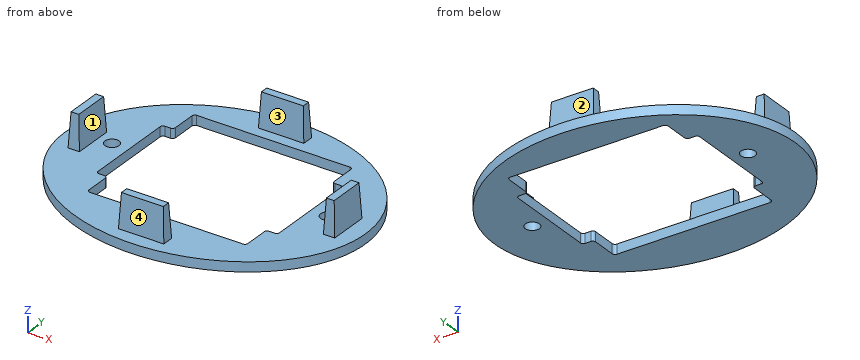
```python
from build123d import *

# Parameters (mm, degrees)
SKETCH1_RX          = 26.5
SKETCH1_RY          = 21.5
SKETCH1_R           = 1.25
BOSS_EXTRUDE1_DEPTH = 1.7
FILLET1_R           = 0.5
SKETCH2_W           = 2
SKETCH2_H           = 7
SKETCH2_W_2         = 8
SKETCH2_H_2         = 2
BOSS_EXTRUDE2_DEPTH = 6
BOSS_EXTRUDE2_TAPER = 3


with BuildPart() as part:
    # Sketch1 → Boss-Extrude1 (new body)
    with BuildSketch(Plane.XY):
        with Locations(Location((0, 0), (0, 0, 180))):
            Ellipse(SKETCH1_RX, SKETCH1_RY)
        with Locations((-19, 1.25)):
            Circle(SKETCH1_R, mode=Mode.SUBTRACT)
        with Locations((19, 1.25)):
            Circle(SKETCH1_R, mode=Mode.SUBTRACT)
        Polygon((-14, 15), (14, 15), (14, 9.75), (16, 9.75), (16, -7.25), (14, -7.25), (14, -12.5), (-14, -12.5), (-14, -7.25), (-16, -7.25), (-16, 9.75), (-14, 9.75), align=None, mode=Mode.SUBTRACT)
    extrude(amount=BOSS_EXTRUDE1_DEPTH)

    # Fillet1
    fillet1_edges = [part.edges().sort_by_distance(p)[0] for p in [
        (-14, 15, 0.85),
        (-14, 9.75, 0.85),
        (-16, 9.75, 0.85),
        (-16, -7.25, 0.85),
        (-14, -7.25, 0.85),
        (-14, -12.5, 0.85),
        (14, -12.5, 0.85),
        (14, -7.25, 0.85),
        (16, -7.25, 0.85),
        (16, 9.75, 0.85),
        (14, 9.75, 0.85),
        (14, 15, 0.85),
    ]]
    fillet(fillet1_edges, radius=FILLET1_R)

    # Sketch2 → Boss-Extrude2 (add)
    with BuildSketch(Plane.XY.offset(1.7)):
        with Locations((-22.5, 0)):
            Rectangle(SKETCH2_W, SKETCH2_H)
        with Locations((0, 18)):
            Rectangle(SKETCH2_W_2, SKETCH2_H_2)
        with Locations((0, -18)):
            Rectangle(SKETCH2_W_2, SKETCH2_H_2)
        with Locations((22.5, 0)):
            Rectangle(SKETCH2_W, SKETCH2_H)
    extrude(amount=BOSS_EXTRUDE2_DEPTH, taper=BOSS_EXTRUDE2_TAPER)


solid = part.part
```
Here's how the part is built. I have some questions about the finished solid (model axes, mm). Face numbers are marked on the shaded views. Give positions to 0.01 mm unless a question says otherwise; leave off trailing zeros. Order: outer loops, then holes, each group sorted by start corner. A loop starts at its lowest first (then second) coordinate and runs counter-clockwise, first axis right, second up. Notation, with made-up numbers: (-11.75, 31) - (-2.75, 31) arc R7 cw to (-2.75, 37) - close; hole circle Ø6 at (20.5, 6). An arc over 180 degrees is marked (long way). Answer as a JSON object with one key per item and string values. Group by question number.
Item 1: If we section it at B-B on y = 1.25: Give the number of separate pieces and of enclosed holes in the cut face, and give its area (3 significant figures).
Item 2: If we section it at C-C on z = 5.5: Please give me the cut outline in (x, y), and give its area (3 significant figures).
Item 3: If we section it at A-A on z = 2.5: Please give me the cut outline in (x, y).
Item 4: Please list where these lines run through material, in increasing order: probe 1 along Y at (x, z) = (2, 7); probe 2 along Z at (x, y) = (-19, -12); probe 3 along Y at (x, z) = (2, 5.75).
Item 5: For P1, Ø3, axis at y = -12, z = 3, coming from the -X side; P2, Ø1.4, axis at x = -3, z = 0.5, coming from the -Y side; P3, Ø0.8, axis at y = -10, z = 1, coming from the +X side, each with a flat end and sliding along its axis, tell me the tip position at first contact or that it passes through.
Item 6: If we mould it in two halves opening along Y, with no side actions, what happens to the marked faces 1, 2, 3 and 4? For each: pulls with the +Y half, pulls with the -Y half, needs draft (parallel to the pull), parting line crosses it, or undercut.
Result set:
{
 "1": {"separate pieces": "4", "enclosed holes": "0", "area": "47.3 mm²"},
 "2": {"outline": "(-23.3, -3.3) - (-21.7, -3.3) - (-21.7, 3.3) - (-23.3, 3.3) - close; (-3.8, -18.8) - (3.8, -18.8) - (3.8, -17.2) - (-3.8, -17.2) - close; (-3.8, 17.2) - (3.8, 17.2) - (3.8, 18.8) - (-3.8, 18.8) - close; (21.7, -3.3) - (23.3, -3.3) - (23.3, 3.3) - (21.7, 3.3) - close", "area": "45.5 mm²"},
 "3": {"outline": "(-23.46, -3.46) - (-21.54, -3.46) - (-21.54, 3.46) - (-23.46, 3.46) - close; (-3.96, -18.96) - (3.96, -18.96) - (3.96, -17.04) - (-3.96, -17.04) - close; (-3.96, 17.04) - (3.96, 17.04) - (3.96, 18.96) - (-3.96, 18.96) - close; (21.54, -3.46) - (23.46, -3.46) - (23.46, 3.46) - (21.54, 3.46) - close"},
 "4": {"probe 1": "-18.72 to -17.28, 17.28 to 18.72", "probe 2": "0 to 1.7", "probe 3": "-18.79 to -17.21, 17.21 to 18.79"},
 "5": {"P1": "x = -22.58", "P2": "y = -21.42", "P3": "x = 23.71"},
 "6": {"face 1": "needs draft", "face 2": "pulls with the +Y half", "face 3": "undercut", "face 4": "pulls with the -Y half"}
}
